```python
from build123d import *

# Parameters (mm, degrees)
SKETCH1_R           = 1
BOSS_EXTRUDE1_DEPTH = 3.6


with BuildPart() as part:
    # Sketch1 → Boss-Extrude1 (new body)
    with BuildSketch(Plane.XY):
        with BuildLine():
            Line((0, 5), (39, 5))
            ThreePointArc((39, 5), (42.984713636, 3.020274365), (43.813971379, -1.351177103))
            Line((43.813971379, -1.351177103), (42.220957068, -7.026765655))
            ThreePointArc((42.220957068, -7.026765655), (33.977057678, -12.429911776), (27.5, -5))
            Line((27.5, -5), (3.651745661, -5))
            Line((3.651745661, -5), (2.3, -10))
            ThreePointArc((2.3, -10), (0, -12.3), (-2.3, -10))
            Line((-2.3, -10), (-4.999999906, -0.00096864))
            ThreePointArc((-4.999999906, -0.00096864), (-3.535876355, 3.535191424), (0, 5))
        make_face()
        with Locations((0, -10)):
            Circle(SKETCH1_R, mode=Mode.SUBTRACT)
        Circle(SKETCH1_R, mode=Mode.SUBTRACT)
        with Locations((39, 0)):
            Circle(SKETCH1_R, mode=Mode.SUBTRACT)
        with Locations((33.8952959, -7.766976867)):
            Circle(SKETCH1_R, mode=Mode.SUBTRACT)
    extrude(amount=BOSS_EXTRUDE1_DEPTH)


solid = part.part
```
CAD build for the part. Positions are in the model's coordinates, mm. A direction names the side the tool comes from. Round coordinates to 2 decimals unless told otherwise and drop trailing zeros. Order: outer loops, then holes, each group sorted by start corner. A loop starts at its lowest first (then second) coordinate and runs counter-clockwise, first axis right, second up.
Q1. Wall check: L1, parallel to X at y = 0.25, z = 2.25; L2, parallel to Y at x = 6, z = 1.3; L3, parallel to X at y = -7.5, z = 1.1. Give the ranges that are in metal, low to high.
Q2. Drop flat-ended pins along their axis: pin 1 (1.2 mm diameter, centred on x = 0, y = -10, fed in from -Z); pin 2 (1.1 mm diameter, centred on x = 13.5, z = 1, fed in from -Y). Give the stop position or say it passes through.
Q3. Two-plate mould, pull along X, no slides. Class faces 3 (the flat face through (2.985, -7.465, 1.775)), 4 (the cylindrical face through (34.13, -12.45, 1.77)), 5 (the cylindrical face through (-4, 3, 2)), 6 (the flat face through (20, -2, 0)): pulls with the +X half, pulls with the -X half, needs draft (parallel to the pull), parting line crosses it, or undercut.
Q4. Slice it at B-B (x = 16.5). Write the cut outline in (y, z).
Q5. Slice it at A-A (z = 1.4). Write the cut outline in (x, y), and give its area (3 significant figures).
Q6. Which spindle directions (+Z, -Z, +X, -X, +Y, -Y) get a long thin tool onto all of the face, cutting with end or side? Do faces 1 (the flat face through (16, -5, 2)), 2 (the flat face through (-3.63, -5.07, 1.77)). Say none if no direction does.
Results below:
1. L1: x = -4.99 to -0.97, 0.97 to 38.03, 39.97 to 43.99
1. L2: y = -5 to 5
1. L3: x = -2.98 to 2.98, 27.93 to 32.93, 34.86 to 42.07
2. pin 1: passes through
2. pin 2: stops at y = -5
3. face 3: undercut
3. face 4: undercut
3. face 5: pulls with the -X half
3. face 6: needs draft
4. outline: (-5, 0) - (5, 0) - (5, 3.6) - (-5, 3.6) - close
5. outline: (-5, 0) - (-2.3, -10) arc R2.3 ccw to (2.3, -10) - (3.65, -5) - (27.5, -5) arc R7.5 ccw to (42.22, -7.03) - (43.81, -1.35) arc R5 ccw to (39, 5) - (0, 5) arc R5 ccw to start; hole circle Ø2 at (0, -10); hole circle Ø2 at (0, 0); hole circle Ø2 at (33.9, -7.77); hole circle Ø2 at (39, 0)
5. area: 587 mm2
6. face 1: +Z, -Z, -Y
6. face 2: +Z, -Z, -X, -Y
